Check sheet for the drawn part. Datum: minimum x, y, z corner. Units: mm. A direction names the side the tool comes from. Give positions to 0.01 mm unless a question says otherwise; leave off trailing zeros. Write each loop counter-clockwise with the first axis right and the second up, starting at its lowest first coordinate (ties: lowest second). Pieces come first, ordered by that corner, then holes. Notation, with made-up numbers: M 49.5,65.25 L 82.5,65.25 A13 cw 82.5,78.25 Z; hole C 17.25,89.5 d7. An arc over 180 degrees is marked long. Write item = value, one per line.
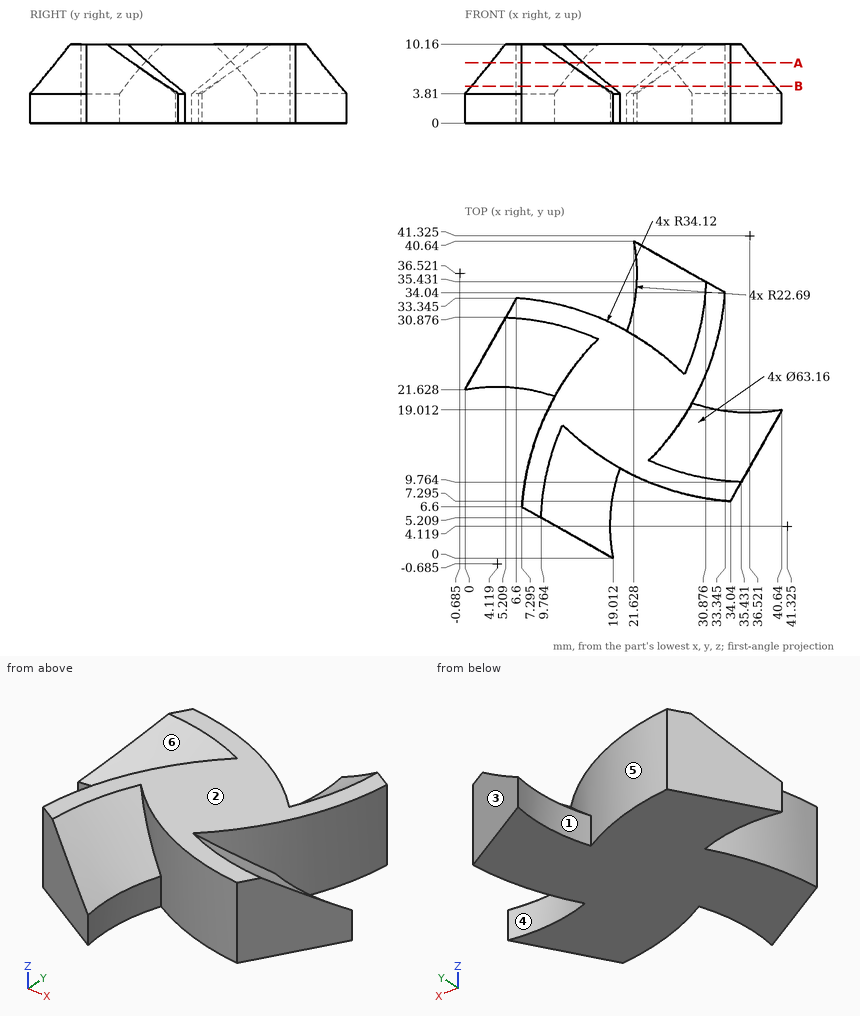
1) Tool access check on the marked faces 4, 5 and 6. Record the directions out of +Z, -Z, +X, -X, +Y, -Y that give a thin tool (end or side, any length) a straight path to the whole face; none if there is none.
From the geometry:
face_4 = +Z, -Z
face_5 = +Z, +Y
face_6 = +Z
2) Cross-section at A-A on z = 7.75. Record the boundary of the cut face in (x, y) (1 decimal), plus the area to 3 significant figures.
From the geometry:
outline = M 3.3,27.5 A28.2 cw 14.7,25.5 A34.1 ccw 7.3,6.6 L 13.1,3.3 A28.2 cw 15.2,14.7 A34.1 ccw 34,7.3 L 37.3,13.1 A28.2 cw 25.9,15.2 A34.1 ccw 33.3,34 L 27.5,37.3 A28.2 cw 25.5,25.9 A34.1 ccw 6.6,33.3 Z
area = 505 mm^2
3) Depth check by flat-ended pin: P1, Ø3, axis at x = 25.5, z = 3, coming from the -Y side. Enter the tip coordinate at first touch or a pass-through.
From the geometry:
P1 = 8.56
4) Material ranges on probe 1 along X at (y, z) = (34.5, 5) (1 decimal); probe 2 along X at (y, z) = (13.5, 9.5) (1 decimal); probe 3 along X at (y, z) = (27, 9.5) (1 decimal), recorded low to high. Write a range as from..to.
From the geometry:
probe_1 = 23.6..32.5
probe_2 = 8.5..12.1, 16.8..24.5
probe_3 = 16..24.1, 28.5..32.1
5) Cross-section at B-B on z = 4.75. Record the boundary of the cut face in (x, y) (1 decimal).
From the geometry:
outline = M 0.8,23.1 A24 cw 12.2,21.9 A34.1 ccw 7.3,6.6 L 17.5,0.8 A24 cw 18.7,12.2 A34.1 ccw 34,7.3 L 39.8,17.5 A24 cw 28.4,18.7 A34.1 ccw 33.3,34 L 23.1,39.8 A24 cw 21.9,28.4 A34.1 ccw 6.6,33.3 Z
6) Draft check along Y on the marked faces 1, 2 and 3. Enter one of: +Y half, -Y half, draft (parallel to the pull), parting line (faces both ways), or undercut.
From the geometry:
face_1 = undercut
face_2 = draft
face_3 = +Y half
